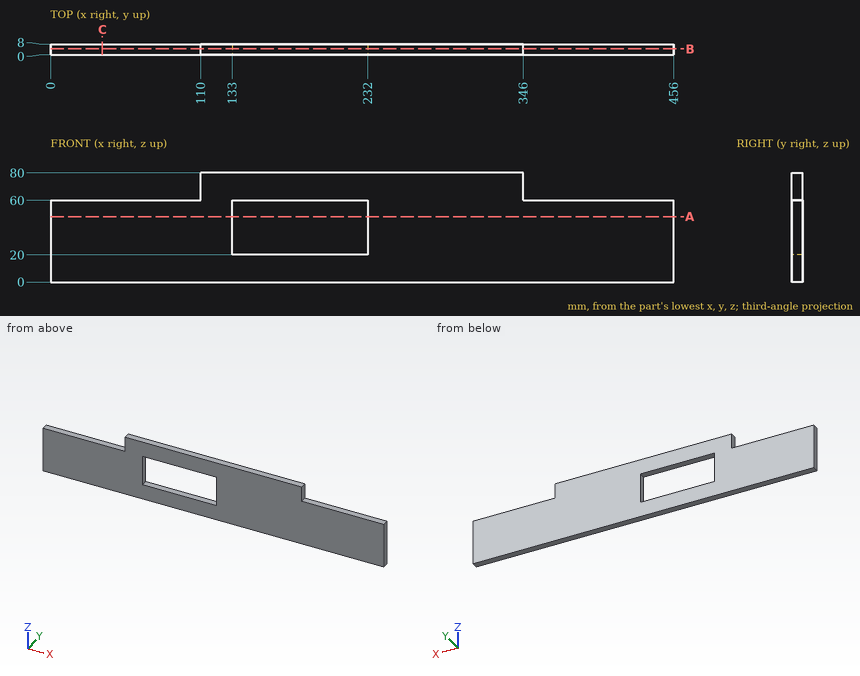
Source: three-view drawing plus pictorial views. Frame: mm from the lowest corner of the part. Give positions to 0.01 mm unless a question says otherwise; leave off trailing zeros. Order: outer loops, then holes, each group sorted by start corner. A loop starts at its lowest first (then second) coordinate and runs counter-clockwise, first axis right, second up. Notation, with made-up numbers: (56, -15.75) -> (75, -15.75) arc R31 ccw to (75, 19.25) -> close; hole circle Ø3 at (9, -39). An arc over 180 degrees is marked (long way). Use a Markdown table: item, result.
Q1. Material intervals for line 1 (X direction, y = 5.5, z = 23); line 2 (Z direction, x = 136, y = 4.75); line 3 (Z direction, x = 99, y = 7.5), sorted ascending. Write a range as [from, to].
A:
| item | result |
|---|---|
| line 1 | [0, 133], [232, 456] |
| line 2 | [0, 20], [60, 80] |
| line 3 | [0, 60] |
Q2. First-contact query: P1, Ø2, axis at y = 2, z = 68, coming from the -X side; P2, Ø2.5, axis at y = 3, z = 73.5, coming from the +X side; P3, Ø4, axis at x = 33.5, y = 4.5, coming from the +Z side. Flat tips, straight axial feed; report the tip coordinate or a pass-through.
A:
| item | result |
|---|---|
| P1 | x = 110 |
| P2 | x = 346 |
| P3 | z = 60 |
Q3. Section C-C (x = 38). Return the cut outline in (y, z), and give its area (3 significant figures).
A:
| item | result |
|---|---|
| outline | (0, 0) -> (8, 0) -> (8, 60) -> (0, 60) -> close |
| area | 480 mm^2 |
Q4. Section B-B (y = 4.5). Return the cut outline in (x, z), and give its area (3 significant figures).
A:
| item | result |
|---|---|
| outline | (0, 0) -> (456, 0) -> (456, 60) -> (346, 60) -> (346, 80) -> (110, 80) -> (110, 60) -> (0, 60) -> close; hole (133, 20) -> (232, 20) -> (232, 60) -> (133, 60) -> close |
| area | 28,100 mm^2 |
Q5. Section A-A (z = 48). Return the cut outline in (x, y).
A:
| item | result |
|---|---|
| outline | (0, 0) -> (133, 0) -> (133, 8) -> (0, 8) -> close; (232, 0) -> (456, 0) -> (456, 8) -> (232, 8) -> close |
